```python
from build123d import *

# Parameters (mm, degrees)
F0_W     = 8
F0_H     = 3
F0_W_2   = 7
F0_H_2   = 5
F0_W_3   = 14
F0_H_3   = 10.4
F1_DEPTH = 2
F2_DEPTH = 5.5


with BuildPart() as f1:
    # F0 (on Top) → F1 (new body)
    with BuildSketch(Plane.XY):
        Polygon((-14.607415, 29.390514), (-14.607415, 37.890514), (-19.707415, 37.890514), (-19.707415, -5.409486), (-10.607415, -5.409486), (-1.507415, -5.409486), (-1.507415, 37.890514), (-6.607415, 37.890514), (-6.607415, 29.390514), (-10.607415, 29.390514), align=None)
        with Locations((-10.607415, 3.790514)):
            Rectangle(F0_W, F0_H, mode=Mode.SUBTRACT)
        with Locations((-10.607415, 12.390514)):
            Rectangle(F0_W_2, F0_H_2, mode=Mode.SUBTRACT)
        with Locations((7.492585, 24.190514)):
            Rectangle(F0_W_3, F0_H_3)
        with BuildLine():
            ThreePointArc((11.242585, 25.940514), (12.480022, 25.427951), (12.992585, 24.190514))
            ThreePointArc((12.992585, 24.190514), (12.480022, 22.953077), (11.242585, 22.440514))
            Line((11.242585, 22.440514), (3.742585, 22.440514))
            ThreePointArc((3.742585, 22.440514), (1.992585, 24.190514), (3.742585, 25.940514))
            Line((3.742585, 25.940514), (11.242585, 25.940514))
        make_face(mode=Mode.SUBTRACT)
        with Locations((-28.707415, 24.190514)):
            Rectangle(F0_W_3, F0_H_3)
        with BuildLine():
            ThreePointArc((-32.457415, 22.440514), (-34.207415, 24.190514), (-32.457415, 25.940514))
            Line((-32.457415, 25.940514), (-24.957415, 25.940514))
            ThreePointArc((-24.957415, 25.940514), (-23.719978, 25.427951), (-23.207415, 24.190514))
            ThreePointArc((-23.207415, 24.190514), (-23.719978, 22.953077), (-24.957415, 22.440514))
            Line((-24.957415, 22.440514), (-32.457415, 22.440514))
        make_face(mode=Mode.SUBTRACT)
    extrude(amount=F1_DEPTH)

    # F0 (on Top) → F2 (join)
    with BuildSketch(Plane.XY):
        Polygon((-19.707415, 37.890514), (-14.607415, 37.890514), (-14.607415, 39.890514), (-21.707415, 39.890514), (-21.707415, 29.390514), (-21.707415, 18.990514), (-21.707415, -7.409486), (-10.607415, -7.409486), (0.492585, -7.409486), (0.492585, 18.990514), (0.492585, 29.390514), (0.492585, 39.890514), (-6.607415, 39.890514), (-6.607415, 37.890514), (-1.507415, 37.890514), (-1.507415, -5.409486), (-10.607415, -5.409486), (-19.707415, -5.409486), align=None)
    extrude(amount=F2_DEPTH)


solid = f1.part
```
The listing builds one solid part. Answer for the finished solid, in the listing's coordinates (mm). A direction names the side the tool comes from. Coordinates: 2 decimals unless noted, no trailing zeros. Write each loop counter-clockwise with the first axis right and the second up, starting at its lowest first coordinate (ties: lowest second). Pieces come first, ordered by that corner, then holes.
Q1. Section C-C, the plane y = 32 is taken. Write down the section's boundary in (x, z).
Returned:
outline: (-21.71, 0) - (-14.61, 0) - (-14.61, 2) - (-19.71, 2) - (-19.71, 5.5) - (-21.71, 5.5) - close; (-6.61, 0) - (0.49, 0) - (0.49, 5.5) - (-1.51, 5.5) - (-1.51, 2) - (-6.61, 2) - close
Q2. The mould has two halves that part along Y. Classify faces 5 (the flat face through (-11, 17, 0)), 6 (the flat face through (-11, 29.391, 1)), 7 (the flat face through (7, 18.991, 1)), 8 (the flat face through (-10, -5.409, 4)): released by +Y, released by -Y, zero draft, split by the parting line, or undercut.
Returned:
face 5: zero draft
face 6: released by +Y
face 7: released by -Y
face 8: undercut
Q3. Section B-B, the plane z = 1.4 is taken. Give the number of separate pieces and of enclosed holes in the cut face, then the cut area to 3 significant figures.
Returned:
separate pieces: 1
enclosed holes: 4
area: 1,130 mm2
Q4. Which of the six approach directions +Z, -Z, +X, -X, +Y, -Y give full straight-line access (tool end or side, diameter ignored) to faces 1 (the flat face through (-17, 37.891, 4)), 2 (the flat face through (-29, 18.991, 1)), 3 (the flat face through (-11, 2.291, 1)), 4 (the flat face through (-14.607, 36, 1))?
Returned:
face 1: +Z
face 2: +Z, -Z, -X, -Y
face 3: +Z, -Z
face 4: +Z, -Z, +Y
Q5. Given P1, Ø1.8, axis at x = -9, z = 4.5, coming from the +Y side; P2, Ø3, axis at y = 32.5, z = 4, coming from the +X side; P3, Ø3, axis at x = -15, y = 2.5, coming from the +Z side, each flat-ended and moving along its own axis, determine where each tip first touches the part or whether it passes through.
Returned:
P1: stops at y = -5.41
P2: stops at x = 0.49
P3: stops at z = 2
Q6. Section A-A, the plane x = 5.5 is taken. Write down the section's boundary in (y, z).
Returned:
outline: (18.99, 0) - (22.44, 0) - (22.44, 2) - (18.99, 2) - close; (25.94, 0) - (29.39, 0) - (29.39, 2) - (25.94, 2) - close
Q7. Find the intervals of material crossed by line 1 along X through (y, z) = (12.5, 3.45); line 2 along Y through (x, z) = (-16, 3.2); line 3 along Y through (x, z) = (-28.5, 0.7), in increasing order.
Returned:
line 1: x = -21.71 to -19.71, -1.51 to 0.49
line 2: y = -7.41 to -5.41, 37.89 to 39.89
line 3: y = 18.99 to 22.44, 25.94 to 29.39
Q8. Section D-D, the plane y = 7.5 is taken. Write down the section's boundary in (x, z), then the cut area to 3 significant figures.
Returned:
outline: (-21.71, 0) - (0.49, 0) - (0.49, 5.5) - (-1.51, 5.5) - (-1.51, 2) - (-19.71, 2) - (-19.71, 5.5) - (-21.71, 5.5) - close
area: 58.4 mm2
